Read the model definition and answer for the solid it produces. Units are mm, in the model's axes. A direction names the side the tool comes from. Round coordinates to 2 decimals unless told otherwise and drop trailing zeros. Write each loop counter-clockwise with the first axis right and the second up, starting at its lowest first coordinate (ties: lowest second). Pieces come first, ordered by that corner, then holes.
from build123d import *

# Parameters (mm, degrees)
STOCK_SPIRALE_ENROUL_E_1_START = -7.5
STOCK_SPIRALE_ENROUL_E_1_DEPTH = 15
BOSS_EXTRU_1_DEPTH             = 15
ENL_V_MAT_EXTRU_1_REACH        = 41.844
ESQUISSE40_R                   = 1.25
ENL_V_MAT_EXTRU_39_DEPTH       = 0.1
ESQUISSE45_R                   = 1.25
ENL_V_MAT_EXTRU_44_DEPTH       = 54.34000069


# Read off the part's stored shape, not the designer's step: Stock-spirale_enroulée-1
with BuildPart() as part:
    # Stock-spirale_enroulée-1 outline → Stock-spirale_enroulée-1 (new body)
    with BuildSketch(Plane.XY.offset(STOCK_SPIRALE_ENROUL_E_1_START)):
        Polygon((-32.409116649, 0), (-14.945224597, 0), (-12.326158681, 5.078291377), (-25.783924084, 12.848135855), (-39.918116919, 19.306194835), (-42.53651187, 14.227557472), align=None)
    extrude(amount=STOCK_SPIRALE_ENROUL_E_1_DEPTH)

    # Esquisse1 → Boss.-Extru.1 (add)
    with BuildSketch(Plane.XY.offset(7.5)):
        Polygon((-42.53651187, 14.227557472), (-32.409116649, 0), (-14.945224597, 0), (-19.987274825, -9.776386321), (-47.576330697, 4.452327735), align=None)
    extrude(amount=-BOSS_EXTRU_1_DEPTH)

    # Enlèv. mat.-Extru.1: up to this plane
    enl_v_mat_extru_1_end = Plane(origin=(-39.918116919, 19.306194835, 7.5), z_dir=(0.8888229444852807, -0.45825077562020095, 0))
    # Esquisse2 → Enlèv. mat.-Extru.1 (cut, up to the surface)
    with BuildSketch(Plane(origin=(-11.805211849, 6.088391881, 0), x_dir=(0, 0, -1), z_dir=(0.8887623928011207, -0.4583682025865522, 0)), mode=Mode.PRIVATE) as enl_v_mat_extru_1_sk1:
        Polygon((-7.5, -9.850415736), (-2.5, -9.850415736), (-6.230461265, -17.850415736), (-7.5, -17.850415736), align=None)
    enl_v_mat_extru_1_tool1 = split(extrude(enl_v_mat_extru_1_sk1.sketch, amount=-ENL_V_MAT_EXTRU_1_REACH, mode=Mode.PRIVATE), bisect_by=enl_v_mat_extru_1_end, keep=Keep.BOTH, mode=Mode.PRIVATE)
    add(enl_v_mat_extru_1_tool1.solids().sort_by_distance((-17.790155, -5.516236, 5.747642))[0], mode=Mode.SUBTRACT)
    # Esquisse2 → Enlèv. mat.-Extru.1 (cut, up to the surface)
    with BuildSketch(Plane(origin=(-11.805211849, 6.088391881, 0), x_dir=(0, 0, -1), z_dir=(0.8887623928011207, -0.4583682025865522, 0)), mode=Mode.PRIVATE) as enl_v_mat_extru_1_sk2:
        Polygon((6.230461265, -17.850415736), (2.5, -9.850415736), (7.5, -9.850415736), (7.5, -17.850415736), align=None)
    enl_v_mat_extru_1_tool2 = split(extrude(enl_v_mat_extru_1_sk2.sketch, amount=-ENL_V_MAT_EXTRU_1_REACH, mode=Mode.PRIVATE), bisect_by=enl_v_mat_extru_1_end, keep=Keep.BOTH, mode=Mode.PRIVATE)
    add(enl_v_mat_extru_1_tool2.solids().sort_by_distance((-17.790155, -5.516236, -5.747642))[0], mode=Mode.SUBTRACT)

    # Esquisse40 → Enlèv. mat.-Extru.39 (cut)
    with BuildSketch(Plane(origin=(-35.583416905, -1.7328691, -7.5), x_dir=(0.8887623928011112, -0.4583682025865705, 0), z_dir=(-0.4583682025865705, -0.8887623928011112, 0))):
        with Locations((-6.504075816, 7.5)):
            Circle(ESQUISSE40_R)
        with Locations((10.556032704, 7.5)):
            Circle(ESQUISSE40_R)
    extrude(amount=-ENL_V_MAT_EXTRU_39_DEPTH, mode=Mode.SUBTRACT)

    # Esquisse45 → Enlèv. mat.-Extru.44 (cut, through all)
    with BuildSketch(Plane(origin=(-8.182062976, -15.864778202, 0), x_dir=(0.8887623928011112, -0.4583682025865705, 0), z_dir=(-0.4583682025865705, -0.8887623928011112, 0))):
        with Locations((-37.334986474, 0)):
            Circle(ESQUISSE45_R)
        with Locations((-20.274877954, 0)):
            Circle(ESQUISSE45_R)
    extrude(amount=-ENL_V_MAT_EXTRU_44_DEPTH, mode=Mode.SUBTRACT)


solid = part.part
Q1. Section C-C (y = 3) is taken. State how many separate pieces and enclosed holes the cut face has, then the cut area to 3 significant figures.
Verdict:
separate pieces: 1
enclosed holes: 2
area: 350 mm2
Q2. Section A-A (z = -3.5) is taken. Determine the outline of the cut face in (x, y).
Verdict:
outline: (-47.58, 4.45) - (-19.99, -9.78) - (-17.3, -4.57) - (-44.89, 9.66) - close; (-43.91, 11.56) - (-16.32, -2.67) - (-12.33, 5.08) - (-25.78, 12.85) - (-39.92, 19.31) - close
Q3. Section B-B (x = -29.5) is taken. Determine the outline of the cut face in (y, z), then the cut area to 3 significant figures.
Verdict:
outline: (-4.87, -6.23) - (4.13, -2.5) - (4.13, -7.5) - (14.55, -7.5) - (14.55, 7.5) - (4.13, 7.5) - (4.13, 2.5) - (-4.87, 6.23) - close
area: 235 mm2
Q4. Determine the mould class of faces 4 (the flat face through (-28, 8, -7.5)), 5 (the flat face through (-18.96, 8.91, -1.77)), 6 (the flat face through (-29.922, 4.349, -4.965)) for opening direction X: pulls with the +X half, pulls with the -X half, needs draft (parallel to the pull), parting line crosses it, or undercut.
Verdict:
face 4: needs draft
face 5: pulls with the +X half
face 6: undercut
Q5. Section D-D (x = -14.5) is taken. Determine the outline of the cut face in (y, z), then the cut area to 3 significant figures.
Verdict:
outline: (0.86, -7.5) - (6.33, -7.5) - (6.33, 7.5) - (0.86, 7.5) - close
area: 82.1 mm2
Q6. Which of the six approach directions +Z, -Z, +X, -X, +Y, -Y give full straight-line access (tool end or side, diameter ignored) to faces 1 (the flat face through (-32.75, 16.03, -1.77)), 2 (the flat face through (-31.781, 0.744, -4.391)), 3 (the flat face through (-31.73, 0.84, 4.34))?
Verdict:
face 1: +Z, -Z, +X, +Y
face 2: -Z
face 3: +Z
Q7. Flat-ended cylindrical pins translate along their axes: pin 1 Ø1.5 at (x, z) = (-34.5, -1.5) entering from +Y; pin 2 Ø4 at (x, z) = (-33.5, -0.5) entering from +Y; pin 3 Ø6 at (x, y) = (-28, -1.5) entering from +Z. Find the tip coordinate at first contact, or state that the pin passes through.
Verdict:
pin 1: stops at y = 17.17
pin 2: stops at y = 17.29
pin 3: stops at z = 5.91
Q8. Straight lines are drawn through the part: probe 1 along Y at (x, z) = (-30.5, -3); probe 2 along Y at (x, z) = (-21.5, -4.5); probe 3 along X at (y, z) = (13.75, -0.5). For each, find the intervals that lie inside material, in ascending order.
Verdict:
probe 1: y = -4.35 to 3.44, 4.65 to 15
probe 2: y = -9 to -4.82, 0.01 to 10.37
probe 3: x = -42.78 to -36.21, -33.63 to -27.76
